Design review of the part built by this model. Coordinates are the model's own, in mm. A direction names the side the tool comes from. Give positions to 0.01 mm unless a question says otherwise; leave off trailing zeros. Write each loop counter-clockwise with the first axis right and the second up, starting at its lowest first coordinate (ties: lowest second). Pieces come first, ordered by that corner, then holes. Notation, with made-up numbers: (-12.75, 47) - (18.25, 47) arc R22 cw to (18.25, 55) - close; hole circle Ø9 at (-35, -40). An arc over 180 degrees is marked (long way). Write each question's results on one line, items separated by ' | '. Start each with the question number.
from build123d import *

# Parameters (mm, degrees)
SKETCH1_R           = 90
SKETCH1_R_2         = 25
BOSS_EXTRUDE1_DEPTH = 3.175
SKETCH2_R           = 2
CUT_EXTRUDE1_DEPTH  = 128.31881489
CUT_EXTRUDE2_DEPTH  = 128.31881489


with BuildPart() as part:
    # Sketch1 → Boss-Extrude1 (new body)
    with BuildSketch(Plane.XY):
        Circle(SKETCH1_R)
        Circle(SKETCH1_R_2, mode=Mode.SUBTRACT)
    extrude(amount=BOSS_EXTRUDE1_DEPTH)

    # Sketch2 → Cut-Extrude1 (cut, through all)
    with BuildSketch(Plane(origin=(0, 0, 0), x_dir=(-1, 0, 0), z_dir=(0, 0, -1))):
        with Locations((-49.523301376, 14.748786792)):
            Circle(SKETCH2_R)
        with Locations((-51.58474767, 4.963571456)):
            Circle(SKETCH2_R)
        with Locations((-37.534474725, -35.514043674)):
            Circle(SKETCH2_R)
        with Locations((-30.09095281, -42.191916202)):
            Circle(SKETCH2_R)
        with Locations((11.988826651, -50.262830467)):
            Circle(SKETCH2_R)
        with Locations((21.493794861, -47.155487659)):
            Circle(SKETCH2_R)
        with Locations((49.523301376, -14.748786792)):
            Circle(SKETCH2_R)
        with Locations((51.58474767, -4.963571456)):
            Circle(SKETCH2_R)
        with Locations((37.534474725, 35.514043674)):
            Circle(SKETCH2_R)
        with Locations((30.09095281, 42.191916202)):
            Circle(SKETCH2_R)
        with Locations((-21.493794861, 47.155487659)):
            Circle(SKETCH2_R)
        with Locations((-11.988826651, 50.262830467)):
            Circle(SKETCH2_R)
    extrude(amount=-CUT_EXTRUDE1_DEPTH, mode=Mode.SUBTRACT)

    # Sketch3 → Cut-Extrude2 (cut, through all)
    with BuildSketch(Plane.XY.offset(3.175)):
        Polygon((-80, 0), (-73.200702677, -32.27471344), (-55.311643355, -28.50603449), (-62.110940678, 3.76867895), align=None)
        with BuildLine():
            Line((-73.200702677, -32.27471344), (-80, 0))
            ThreePointArc((-80, 0), (-78.281722688, -16.49157036), (-73.200702677, -32.27471344))
        make_face()
        with BuildLine():
            Line((-59.849640055, 4.245065992), (-62.110940678, 3.76867895))
            Line((-62.110940678, 3.76867895), (-58.711292321, -12.368676325))
            ThreePointArc((-58.711292321, -12.368676325), (-59.859650683, -4.101489986), (-59.849640055, 4.245065992))
        make_face()
        with BuildLine():
            ThreePointArc((-53.050342732, -28.029647448), (-56.426786826, -20.396512655), (-58.711292321, -12.368676325))
            Line((-58.711292321, -12.368676325), (-55.311643355, -28.50603449))
            Line((-55.311643355, -28.50603449), (-53.050342732, -28.029647448))
        make_face()
        Polygon((-34.319242049, -51.905313005), (-2.968871648, -62.154305515), (-8.649629599, -79.531024813), (-40, -69.282032303), align=None)
        with BuildLine():
            Line((-33.601155018, -49.708775699), (-34.319242049, -51.905313005))
            Line((-34.319242049, -51.905313005), (-18.644036991, -57.029815752))
            ThreePointArc((-18.644036991, -57.029815752), (-26.377820776, -53.890728063), (-33.601155018, -49.708775699))
        make_face()
        with BuildLine():
            ThreePointArc((-2.250784617, -59.957768209), (-10.549484296, -59.065289139), (-18.644036991, -57.029815752))
            Line((-18.644036991, -57.029815752), (-2.968871648, -62.154305515))
            Line((-2.968871648, -62.154305515), (-2.250784617, -59.957768209))
        make_face()
        with BuildLine():
            Line((-8.649629599, -79.531024813), (-40, -69.282032303))
            ThreePointArc((-40, -69.282032303), (-24.858742464, -76.03974568), (-8.649629599, -79.531024813))
        make_face()
        Polygon((27.791698629, -55.673991955), (52.342771707, -33.648271025), (64.551073077, -47.256311373), (40, -69.282032303), align=None)
        with BuildLine():
            Line((26.248485037, -53.953841691), (27.791698629, -55.673991955))
            Line((27.791698629, -55.673991955), (40.067235173, -44.661131486))
            ThreePointArc((40.067235173, -44.661131486), (33.481820478, -49.789232747), (26.248485037, -53.953841691))
        make_face()
        with BuildLine():
            ThreePointArc((50.799558115, -31.928120761), (45.877291999, -38.668773951), (40.067235173, -44.661131486))
            Line((40.067235173, -44.661131486), (52.342771707, -33.648271025))
            Line((52.342771707, -33.648271025), (50.799558115, -31.928120761))
        make_face()
        with BuildLine():
            Line((64.551073077, -47.256311373), (40, -69.282032303))
            ThreePointArc((40, -69.282032303), (53.422980224, -59.54817532), (64.551073077, -47.256311373))
        make_face()
        Polygon((62.110940678, -3.76867895), (55.311643355, 28.50603449), (73.200702677, 32.27471344), (80, 0), align=None)
        with BuildLine():
            Line((58.711292095, 12.368677398), (55.311643355, 28.50603449))
            Line((55.311643355, 28.50603449), (53.050342732, 28.029647448))
            ThreePointArc((53.050342732, 28.029647448), (56.42678664, 20.39651317), (58.711292095, 12.368677398))
        make_face()
        with BuildLine():
            Line((59.849640055, -4.245065992), (62.110940678, -3.76867895))
            Line((62.110940678, -3.76867895), (58.711292095, 12.368677398))
            ThreePointArc((58.711292095, 12.368677398), (59.676953364, 6.217816108), (60, 0))
            ThreePointArc((60, 0), (59.962398231, -2.123864014), (59.849640055, -4.245065992))
        make_face()
        with BuildLine():
            ThreePointArc((80, 0), (78.281722688, 16.49157036), (73.200702677, 32.27471344))
            Line((73.200702677, 32.27471344), (80, 0))
        make_face()
        Polygon((-27.791698629, 55.673991955), (-52.342771707, 33.648271025), (-64.551073077, 47.256311373), (-40, 69.282032303), align=None)
        Polygon((34.319242049, 51.905313005), (2.968871648, 62.154305515), (8.649629599, 79.531024813), (40, 69.282032303), align=None)
        with BuildLine():
            Line((18.644056811, 57.029809272), (2.968871648, 62.154305515))
            Line((2.968871648, 62.154305515), (2.250784617, 59.957768209))
            ThreePointArc((2.250784617, 59.957768209), (10.54949456, 59.065287306), (18.644056811, 57.029809272))
        make_face()
        with BuildLine():
            Line((33.601155018, 49.708775699), (34.319242049, 51.905313005))
            Line((34.319242049, 51.905313005), (18.644056811, 57.029809272))
            ThreePointArc((18.644056811, 57.029809272), (26.37783014, 53.890723479), (33.601155018, 49.708775699))
        make_face()
        with BuildLine():
            ThreePointArc((40, 69.282032303), (24.858742464, 76.03974568), (8.649629599, 79.531024813))
            Line((8.649629599, 79.531024813), (40, 69.282032303))
        make_face()
        with BuildLine():
            ThreePointArc((-40, 69.282032303), (-53.422980224, 59.54817532), (-64.551073077, 47.256311373))
            Line((-64.551073077, 47.256311373), (-40, 69.282032303))
        make_face()
        with BuildLine():
            Line((-40.067234967, 44.661131671), (-52.342771707, 33.648271025))
            Line((-52.342771707, 33.648271025), (-50.799558115, 31.928120761))
            ThreePointArc((-50.799558115, 31.928120761), (-45.877291909, 38.668774057), (-40.067234967, 44.661131671))
        make_face()
        with BuildLine():
            Line((-26.248485037, 53.953841691), (-27.791698629, 55.673991955))
            Line((-27.791698629, 55.673991955), (-40.067234967, 44.661131671))
            ThreePointArc((-40.067234967, 44.661131671), (-33.481820363, 49.789232824), (-26.248485037, 53.953841691))
        make_face()
    extrude(amount=-CUT_EXTRUDE2_DEPTH, mode=Mode.SUBTRACT)


solid = part.part
Q1. Machinability: for faces 1 (the face through (-53.25, 59.703, 1.61)), 2 (the face through (19, -19, 0)), which of the approach directions +Z, -Z, +X, -X, +Y, -Y give a long, thin tool a straight path to every point of the face, cutting with its end or side? Answer none if there is none.
Q2. Add section A-A on x = 0. State the section outline as (y, z) points (3 decimals), plus the area to 3 significant figures.
Q3. The part is to be moulded in two halves that separate along X. For faces 3 (the face through (23.846, 7.509, 1.565)), 4 (the face through (19, -19, 3.175)), 5 (the face through (29.168, -43.966, 1.565)), 6 (the face through (41.53, -79.845, 1.565)), say which applies: +X half, -X half, draft (parallel to the pull), parting line (faces both ways), or undercut.
Q4. Add section C-C on z = 2.45. Count the separate pieces of the cut face and the enclosed holes in it, plus the area to 3 significant figures.
Q5. Add section D-D on x = -70. State the section outline as (y, z) points (3 decimals), plus the area to 3 significant figures.
Q6. Add section B-B on y = 22.5. State the section outline as (x, z) points (3 decimals).
Q7. Insertion check: P1, Ø3, axis at x = -49.52, y = -14.75, coming from the +Z side (3 decimals). The pin has a flat end and moves straight along its axis. Give the tip position at first contact, or say it passes through.
Q8. For line 1 along Y through (x, z) = (-62, 2.6); line 2 along X through (y, z) = (20, 1.1); line 3 along X through (y, z) = (14.5, 1.4), list the stretches that pass through material, from the lowest coordinate up. Write a range as [from, to].
Result:
1) face 1: +Z, -Z | face 2: -Z, +X, -X, +Y, -Y
2) outline: (-90, 0) - (-25, 0) - (-25, 3.175) - (-90, 3.175) - close; (25, 0) - (90, 0) - (90, 3.175) - (25, 3.175) - close | area: 413 mm²
3) face 3: undercut | face 4: draft | face 5: undercut | face 6: parting line
4) separate pieces: 1 | enclosed holes: 19 | area: 19,300 mm²
5) outline: (-56.569, 0) - (-31.6, 0) - (-31.6, 3.175) - (-56.569, 3.175) - close; (2.107, 0) - (56.569, 0) - (56.569, 3.175) - (2.107, 3.175) - close | area: 252 mm²
6) outline: (-87.142, 0) - (-10.897, 0) - (-10.897, 3.175) - (-87.142, 3.175) - close; (10.897, 0) - (55.621, 0) - (55.621, 3.175) - (10.897, 3.175) - close; (76.771, 0) - (87.142, 0) - (87.142, 3.175) - (76.771, 3.175) - close
7) P1: passes through
8) line 1: y = [-65.24, -29.92], [3.79, 44.41], [50.56, 65.24] | line 2: x = [-87.75, -15], [15, 56.57], [77.46, 87.75] | line 3: x = [-88.82, -20.37], [20.37, 47.54], [51.51, 58.22], [78.67, 88.82]
